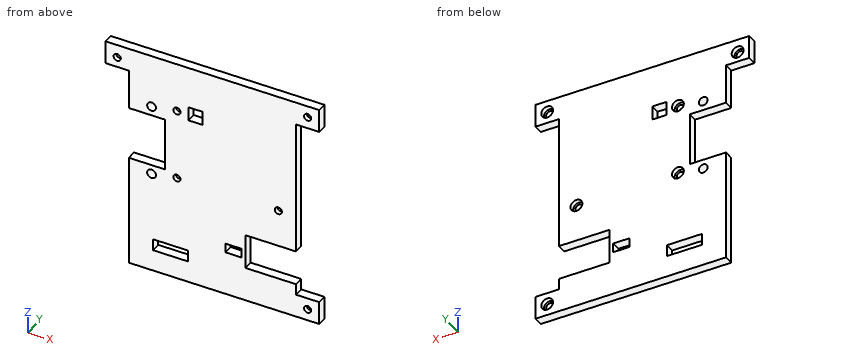
from build123d import *

# Parameters (mm, degrees)
SKETCH1_R           = 0.775
SKETCH1_R_2         = 0.95
SKETCH1_W           = 3
SKETCH1_H           = 3
SKETCH1_W_2         = 3.5
SKETCH1_H_2         = 2
SKETCH1_W_3         = 7.5
SKETCH1_H_3         = 2.5
BOSS_EXTRUDE1_DEPTH = 2
SKETCH2_R           = 1.275
CUT_EXTRUDE1_DEPTH  = 1
SKETCH4_W           = 22.039842778
SKETCH4_H           = 2
SKETCH4_W_2         = 11.560157222
BOSS_EXTRUDE3_DEPTH = 2
SKETCH5_W           = 5.4
SKETCH5_H           = 2
SKETCH5_W_2         = 32.1
BOSS_EXTRUDE4_DEPTH = 2
SKETCH6_W           = 36
SKETCH6_H           = 2
BOSS_EXTRUDE5_DEPTH = 2
SKETCH7_W           = 36
SKETCH7_H           = 2
BOSS_EXTRUDE6_DEPTH = 2
SKETCH8_W           = 5
SKETCH8_H           = 2
BOSS_EXTRUDE7_DEPTH = 5
SKETCH9_W           = 5
SKETCH9_H           = 2
BOSS_EXTRUDE8_DEPTH = 5
SKETCH10_R          = 0.775
CUT_EXTRUDE2_DEPTH  = 5
SKETCH11_R          = 1.275
CUT_EXTRUDE3_DEPTH  = 1


with BuildPart() as part:
    # Sketch1 → Boss-Extrude1 (new body)
    with BuildSketch(Plane(origin=(0, 0, 0), x_dir=(1, 0, 0), z_dir=(0, 1, 0))):
        Polygon((32.485414634, 9.09397561), (23.585414634, 9.09397561), (23.585414634, 1.59397561), (32.485414634, 1.59397561), (32.485414634, -30.50602439), (0.485414634, -30.50602439), (0.485414634, -18.945867168), (6.285414634, -18.945867168), (6.285414634, -7.545867168), (0.485414634, -7.545867168), (0.485414634, 14.49397561), (32.485414634, 14.49397561), align=None)
        with Locations((30.685414634, -6.43902439)):
            Circle(SKETCH1_R, mode=Mode.SUBTRACT)
        with Locations((8.841414634, -6.43902439)):
            Circle(SKETCH1_R, mode=Mode.SUBTRACT)
        with Locations((8.841414634, -21.80602439)):
            Circle(SKETCH1_R, mode=Mode.SUBTRACT)
        with Locations((3.385414634, -5.545867168)):
            Circle(SKETCH1_R_2, mode=Mode.SUBTRACT)
        with Locations((3.385414634, -20.945867168)):
            Circle(SKETCH1_R_2, mode=Mode.SUBTRACT)
        with Locations((12.841414634, -22.013272234)):
            Rectangle(SKETCH1_W, SKETCH1_H, mode=Mode.SUBTRACT)
        with Locations((21.035414634, 5.99397561)):
            Rectangle(SKETCH1_W_2, SKETCH1_H_2, mode=Mode.SUBTRACT)
        with Locations((7.439637151, 10.59397561)):
            Rectangle(SKETCH1_W_3, SKETCH1_H_3, mode=Mode.SUBTRACT)
    extrude(amount=BOSS_EXTRUDE1_DEPTH)

    # Sketch2 → Cut-Extrude1 (cut)
    with BuildSketch(Plane(origin=(0, 2, 0), x_dir=(1, 0, 0), z_dir=(0, 1, 0))):
        with Locations((8.841414634, -6.43902439)):
            Circle(SKETCH2_R)
        with Locations((30.685414634, -6.43902439)):
            Circle(SKETCH2_R)
        with Locations((8.841414634, -21.80602439)):
            Circle(SKETCH2_R)
    extrude(amount=-CUT_EXTRUDE1_DEPTH, mode=Mode.SUBTRACT)

    # Sketch4 → Boss-Extrude3 (add)
    with BuildSketch(Plane.ZY.offset(-0.485414634)):
        with Locations((-3.474054221, 1)):
            Rectangle(SKETCH4_W, SKETCH4_H)
        with Locations((24.725945779, 1)):
            Rectangle(SKETCH4_W_2, SKETCH4_H)
    extrude(amount=BOSS_EXTRUDE3_DEPTH)

    # Sketch5 → Boss-Extrude4 (add)
    with BuildSketch(Plane(origin=(32.485414634, 0, 0), x_dir=(0, 0, -1), z_dir=(1, 0, 0))):
        with Locations((11.79397561, 1)):
            Rectangle(SKETCH5_W, SKETCH5_H)
        with Locations((-14.45602439, 1)):
            Rectangle(SKETCH5_W_2, SKETCH5_H)
    extrude(amount=BOSS_EXTRUDE4_DEPTH)

    # Sketch6 → Boss-Extrude5 (add)
    with BuildSketch(Plane(origin=(0, 0, -14.49397561), x_dir=(-1, 0, 0), z_dir=(0, 0, -1))):
        with Locations((-16.485414634, 1)):
            Rectangle(SKETCH6_W, SKETCH6_H)
    extrude(amount=BOSS_EXTRUDE5_DEPTH)

    # Sketch7 → Boss-Extrude6 (add)
    with BuildSketch(Plane.XY.offset(30.50602439)):
        with Locations((16.485414634, 1)):
            Rectangle(SKETCH7_W, SKETCH7_H)
    extrude(amount=BOSS_EXTRUDE6_DEPTH)

    # Sketch8 → Boss-Extrude7 (add)
    with BuildSketch(Plane(origin=(34.485414634, 0, 0), x_dir=(0, 0, -1), z_dir=(1, 0, 0))):
        with Locations((13.99397561, 1)):
            Rectangle(SKETCH8_W, SKETCH8_H)
        with Locations((-30.00602439, 1)):
            Rectangle(SKETCH8_W, SKETCH8_H)
    extrude(amount=BOSS_EXTRUDE7_DEPTH)

    # Sketch9 → Boss-Extrude8 (add)
    with BuildSketch(Plane.ZY.offset(1.514585366)):
        with Locations((30.00602439, 1)):
            Rectangle(SKETCH9_W, SKETCH9_H)
    extrude(amount=BOSS_EXTRUDE8_DEPTH)

    # Sketch10 → Cut-Extrude2 (cut)
    with BuildSketch(Plane(origin=(0, 2, 0), x_dir=(1, 0, 0), z_dir=(0, 1, 0))):
        with Locations((36.985414634, 13.99397561)):
            Circle(SKETCH10_R)
        with Locations((36.985414634, -30.00602439)):
            Circle(SKETCH10_R)
        with Locations((-4.014585366, -29.691233116)):
            Circle(SKETCH10_R)
    extrude(amount=-CUT_EXTRUDE2_DEPTH, mode=Mode.SUBTRACT)

    # Sketch11 → Cut-Extrude3 (cut)
    with BuildSketch(Plane(origin=(0, 2, 0), x_dir=(1, 0, 0), z_dir=(0, 1, 0))):
        with Locations((36.985414634, 13.99397561)):
            Circle(SKETCH11_R)
        with Locations((36.985414634, -30.00602439)):
            Circle(SKETCH11_R)
        with Locations((-4.014585366, -29.691233116)):
            Circle(SKETCH11_R)
    extrude(amount=-CUT_EXTRUDE3_DEPTH, mode=Mode.SUBTRACT)


solid = part.part
For this review, take the finished solid that the model builds, in its own axes (mm). Give positions to 0.01 mm unless a question says otherwise; leave off trailing zeros. Loops run counter-clockwise (first coordinate to the right, second up) from the corner with the lowest first, then second, coordinate; pieces in that order, holes last. Notation, with made-up numbers: (60.5, -18.5) -> (67.5, -18.5) arc R11 cw to (67.5, -8.5) -> close; hole circle Ø2 at (-34.75, 9.5). An arc over 180 degrees is marked (long way). One line per question, with ' | ' between items.
1) Insertion check: pin 1 Ø2 at (x, z) = (3.39, 20.95) entering from +Y; pin 2 Ø0.6 at (y, z) = (1, -6.5) entering from +X; pin 3 Ø1 at (x, y) = (-4, 0.5) entering from -Z. Each pin has a flat end and moves straight along its axis. Give the tip position at first contact, or say it passes through.
Resolved:
pin 1: stops at y = 2 | pin 2: stops at x = 23.59 | pin 3: stops at z = 27.51
2) We need section C-C (y = 0.5). Give the number of separate pieces and of enclosed holes in the cut face, plus the area to 3 significant figures.
Resolved:
separate pieces: 1 | enclosed holes: 11 | area: 1,620 mm2
3) We need section B-B (z = 1.5). Write out the cut boundary in (x, y), plus the area to 3 significant figures.
Resolved:
outline: (-1.51, 0) -> (34.49, 0) -> (34.49, 2) -> (-1.51, 2) -> close | area: 72.0 mm2
4) We need section A-A (x = 9). Write out the cut boundary in (y, z).
Resolved:
outline: (0, -16.49) -> (2, -16.49) -> (2, -11.84) -> (0, -11.84) -> close; (0, -9.34) -> (2, -9.34) -> (2, 5.17) -> (1, 5.17) -> (1, 5.68) -> (0, 5.68) -> close; (0, 7.2) -> (1, 7.2) -> (1, 7.7) -> (2, 7.7) -> (2, 20.54) -> (1, 20.54) -> (1, 21.05) -> (0, 21.05) -> close; (0, 22.56) -> (1, 22.56) -> (1, 23.07) -> (2, 23.07) -> (2, 32.51) -> (0, 32.51) -> close
5) We need section D-D (z = 18). Write out the cut boundary in (x, y).
Resolved:
outline: (6.29, 0) -> (34.49, 0) -> (34.49, 2) -> (6.29, 2) -> close
6) To check wall thickness, follow probe 1 along Z at (x, y) = (5, 1.7); probe 2 along X at (y, z) = (1.2, 5.5); probe 3 along Z at (x, y) = (25, 1). State the ranges of each line that lie inside material, in increasing order.
Resolved:
probe 1: z = -16.49 to -11.84, -9.34 to 7.55, 18.95 to 32.51 | probe 2: x = -1.51 to 2.44, 4.33 to 7.98, 9.7 to 29.82, 31.55 to 34.49 | probe 3: z = -16.49 to -9.09, -1.59 to 32.51
